Read the model definition and answer for the solid it produces. Units are mm, in the model's axes. Face numbers are marked on the shaded views. A direction names the side the tool comes from. Coordinates: 2 decimals unless noted, no trailing zeros. Write each loop counter-clockwise with the first axis right and the second up, starting at its lowest first coordinate (ties: lowest second). Pieces come first, ordered by that corner, then holes.
(1) Given pin 1 (19.5 mm diameter, centred on x = -32.5, z = 35, fed in from +Y); pin 2 (8 mm diameter, centred on y = -45, z = 40, fed in from +X); pin 3 (22 mm diameter, centred on y = 12, z = 5.5, fed in from -X), each flat-ended and moving along its own axis, determine where each tip first touches the part or whether it passes through.
(2) Straight lines are drawn through the part: line 1 along X through (y, z) = (-43.5, 35); line 2 along Z through (x, y) = (-32, -44); line 3 along Y through (x, z) = (-24, 22). For each, find the intervals that lie inside material, in ascending order.
(3) Which of the six approach directions +Z, -Z, +X, -X, +Y, -Y give full straight-line access (tool end or side, diameter ignored) to the marked faces 4, 5, 6, 7 and 8?
(4) Determine the mould class of the marked faces 1, 2 and 3 for opening direction Z: pulls with the +Z half, pulls with the -Z half, needs draft (parallel to the pull), parting line crosses it, or undercut.
(5) The part is cut by section B-B, the plane z = 41. Determine the outline of the cut face in (x, y), and give its area (3 significant figures).
(6) The part is cut by section C-C, the plane z = 35. Determine the outline of the cut face in (x, y), and give its area (3 significant figures).
(7) The part is cut by section A-A, the plane x = -32.5. Determine the outline of the cut face in (y, z).
(8) The part is cut by section D-D, the plane y = 29. Determine the outline of the cut face in (x, z), and give its area (3 significant figures).
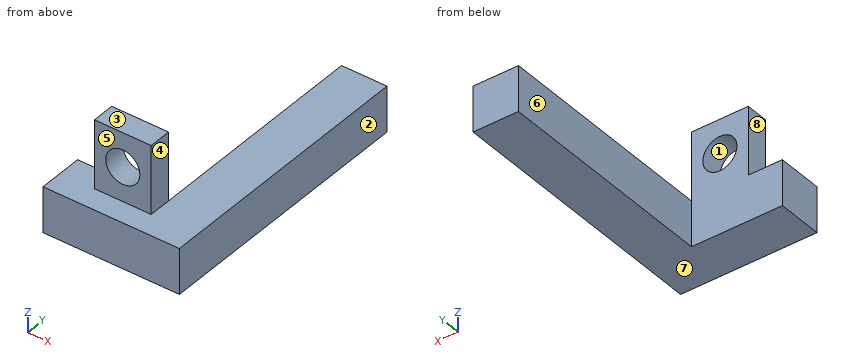
Autodesk Inventor part; units mm, degrees
ref_plane "YZ Plane" through (0, 0, 0) normal (1, 0, 0) x (0, 1, 0)
ref_plane "XZ Plane" through (0, 0, 0) normal (0, 1, 0) x (-1, 0, 0)
ref_plane "XY Plane" through (0, 0, 0) normal (0, 0, 1) x (1, 0, 0)
sketch "Sketch1" plane through (0, 0, 0) normal (0, 0, 1) x (1, 0, 0)
  line L0 (0, 60) -> (0, -60)
  line L1 (0, 60) -> (-20, 60)
  line L2 (-20, 60) -> (-20, -40)
  line L3 (-20, -40) -> (-60, -40)
  line L4 (-60, -40) -> (-60, -60)
  line L5 (-60, -60) -> (0, -60)
  point P0 (0, 0)
  dimension "d0" = 120
  dimension "d1" = 20
  dimension "d2" = 100
  dimension "d3" = 40
  dimension "d4" = 20
extrude "Extrusion1" add sketch "Sketch1" along normal blind 20
sketch "Sketch2" plane through (0, 0, 20) normal (0, 0, 1) x (1, 0, 0)
  line L0 (-20, -40) -> (-60, -40)
  line L1 (-20, -40) -> (-20, -50)
  line L2 (-20, -50) -> (-45, -50)
  line L3 (-45, -50) -> (-45, -40)
  point P0 (0, 0)
  dimension "d7" = 10
  dimension "d8" = 25
extrude "Extrusion2" add sketch "Sketch2" along normal blind 30
sketch "Sketch3" plane through (-60, -40, 0) normal (0, 1, 0) x (1, 0, 0)
  point P0 (60, 0)
sketch "Sketch4" plane through (-60, -40, 0) normal (0, 1, 0) x (1, 0, 0)
  line L0 (40, -50) -> (15, -50)
  line L1 (40, -20) -> (40, -50)
  circle A0 centre (27.5, -35) radius 7.5
  point P0 (60, 0)
  dimension "d11" = 15
extrude "Extrusion3" cut sketch "Sketch4" against normal blind 10
properties part number "steering_helper_base[1]"
Computed:
1. pin 1: stops at y = -40
1. pin 2: stops at x = -20
1. pin 3: stops at x = -20
2. line 1: x = -45 to -40, -25 to -20
2. line 2: z = 0 to 27.52, 42.48 to 50
2. line 3: y = -50 to -40
3. face 4: +Z, +X, +Y, -Y
3. face 5: +Z, +X, -X, -Y
3. face 6: +Z, -Z, -X, +Y
3. face 7: -Z, +X, -X, +Y, -Y
3. face 8: +Z, -X, +Y, -Y
4. face 1: undercut
4. face 2: needs draft
4. face 3: pulls with the +Z half
5. outline: (-45, -50) - (-37, -50) - (-37, -40) - (-45, -40) - close; (-28, -50) - (-20, -50) - (-20, -40) - (-28, -40) - close
5. area: 160 mm2
6. outline: (-45, -50) - (-40, -50) - (-40, -40) - (-45, -40) - close; (-25, -50) - (-20, -50) - (-20, -40) - (-25, -40) - close
6. area: 100 mm2
7. outline: (-60, 0) - (-40, 0) - (-40, 27.5) - (-50, 27.5) - (-50, 20) - (-60, 20) - close; (-50, 42.5) - (-40, 42.5) - (-40, 50) - (-50, 50) - close
8. outline: (-20, 0) - (0, 0) - (0, 20) - (-20, 20) - close
8. area: 400 mm2
